Design review of the part shown in the three views and the two pictorial views. Dimensions are in mm from the part's minimum x, y and z. A direction names the side the tool comes from. Give positions to 0.01 mm unless a question says otherwise; leave off trailing zeros. Loops run counter-clockwise (first coordinate to the right, second up) from the corner with the lowest first, then second, coordinate; pieces in that order, holes last.
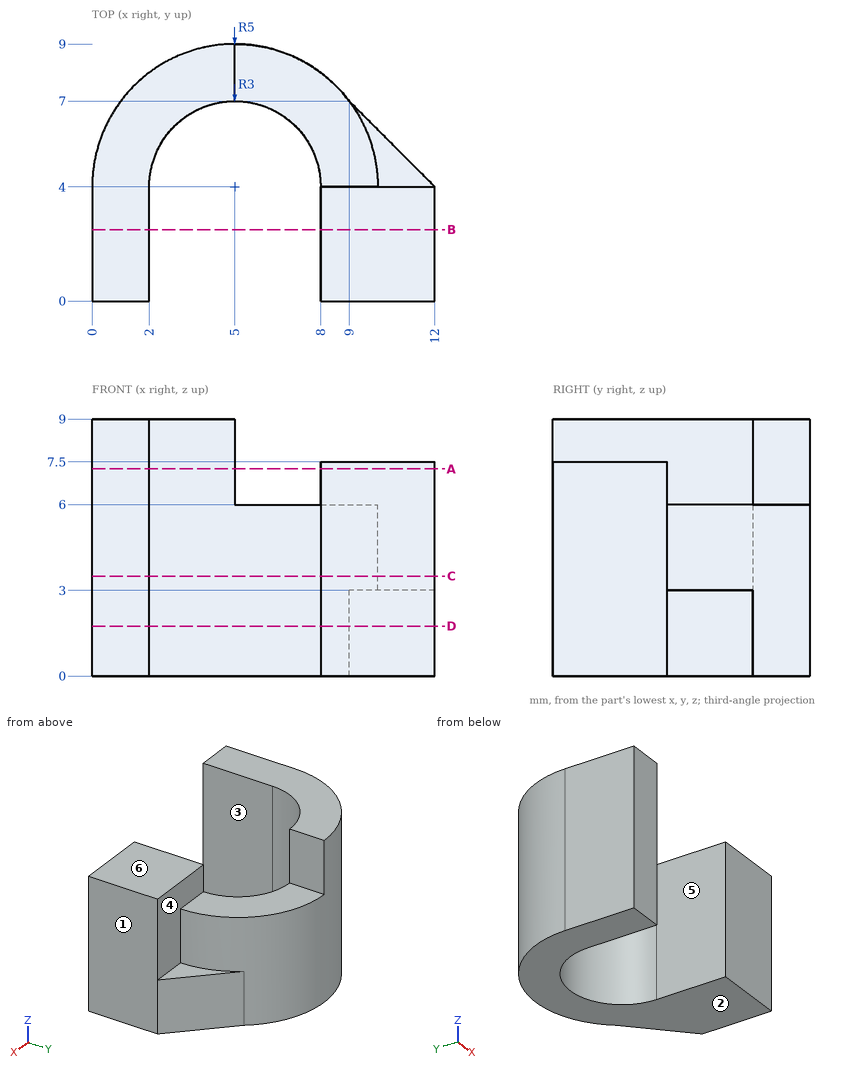
Q1. For pin 1 Ø2 at (y, z) = (7.5, 4.5) entering from +X; pin 2 Ø3 at (x, y) = (10, 2) entering from +Z; pin 3 Ø1 at (x, y) = (3.5, 5) entering from -Z; pin 4 Ø1.2 at (x, z) = (10, 5) entering from +Y, all flat-tipped, find the tip position at first contact; note any pin that passes through.
Answers:
pin 1: stops at x = 9.33
pin 2: stops at z = 7.5
pin 3: passes through
pin 4: stops at y = 6.37
Q2. Machinability: for the marked faces 4, 5 and 6, which of the approach directions +Z, -Z, +X, -X, +Y, -Y give a long, thin tool a straight path to every point of the face, cutting with its end or side? Answer none if there is none.
Answers:
face 4: +Z, +X, +Y
face 5: +Z, -Z, -Y
face 6: +Z, +X, +Y, -Y
Q3. For probe 1 along X at (y, z) = (1.5, 3); probe 2 along X at (y, z) = (6.5, 2); probe 3 along X at (y, z) = (8, 2.75), list the stretches that pass through material, from the lowest coordinate up.
Answers:
probe 1: x = 0 to 2, 8 to 12
probe 2: x = 0.67 to 3.34, 6.66 to 9.5
probe 3: x = 2 to 8
Q4. Consider section A-A on z = 7.25. Give the boundary of the cut face in (x, y).
Answers:
outline: (0, 0) - (2, 0) - (2, 4) arc R3 cw to (5, 7) - (5, 9) arc R5 ccw to (0, 4) - close; (8, 0) - (12, 0) - (12, 4) - (8, 4) - close
Q5. Consider section C-C on z = 3.5. Give the boundary of the cut face in (x, y), plus the area to 3 significant figures.
Answers:
outline: (0, 0) - (2, 0) - (2, 4) arc R3 cw to (8, 4) - (8, 0) - (12, 0) - (12, 4) - (10, 4) arc R5 ccw to (0, 4) - close
area: 49.1 mm2
Q6. Consider section B-B on y = 2.5. Give the boundary of the cut face in (x, z), plus the area to 3 significant figures.
Answers:
outline: (0, 0) - (2, 0) - (2, 9) - (0, 9) - close; (8, 0) - (12, 0) - (12, 7.5) - (8, 7.5) - close
area: 48.0 mm2
Q7. Mouldability with a two-part tool opening along X and no side actions: class the marked faces 1, 2 and 3 as +X half, -X half, draft (parallel to the pull), parting line (faces both ways), or undercut.
Answers:
face 1: +X half
face 2: draft
face 3: undercut
Q8. Consider section D-D on z = 1.75. Give the boundary of the cut face in (x, y).
Answers:
outline: (0, 0) - (2, 0) - (2, 4) arc R3 cw to (8, 4) - (8, 0) - (12, 0) - (12, 4) - (9, 7) arc R5 ccw to (0, 4) - close
